Can you work these out from the model? Positions are in its coordinate system, mm. Give positions to 0.01 mm unless a question says otherwise; leave off trailing zeros. Order: outer loops, then holes, each group sorted by start corner. A loop starts at its lowest first (then second) coordinate and runs counter-clockwise, first axis right, second up. Notation, with made-up numbers: (44, 54) -> (70, 54) arc R36 cw to (70, 91) -> close; hole circle Ø3 at (61.25, 31.5). An arc over 180 degrees is marked (long way). Answer as a JSON object with one key per item and string values.
```python
from build123d import *

# Parameters (mm, degrees)
F0_W     = 25.4
F0_H     = 45.72
F0_W_2   = 6.35
F0_H_2   = 10.0076
F1_DEPTH = 3.175


with BuildPart() as f1:
    # F0 (on Top) → F1 (new body)
    with BuildSketch(Plane.XY):
        Polygon((-45.72, 76.2), (-76.2, 76.2), (-76.2, 45.72), (-73.025, 45.72), (-73.025, 15.24), (-76.2, 15.24), (-76.2, -15.24), (-73.025, -15.24), (-73.025, -45.72), (-76.2, -45.72), (-76.2, -76.2), (-45.72, -76.2), (-45.72, -73.025), (-15.24, -73.025), (-15.24, -76.2), (15.24, -76.2), (15.24, -73.025), (45.72, -73.025), (45.72, -76.2), (76.2, -76.2), (76.2, -45.72), (73.025, -45.72), (73.025, -15.24), (76.2, -15.24), (76.2, 15.24), (73.025, 15.24), (73.025, 45.72), (76.2, 45.72), (76.2, 76.2), (45.72, 76.2), (45.72, 73.025), (15.24, 73.025), (15.24, 76.2), (-15.24, 76.2), (-15.24, 73.025), (-45.72, 73.025), align=None)
        with Locations((-38.1, -38.1)):
            Rectangle(F0_W, F0_H, mode=Mode.SUBTRACT)
        with Locations((0, -38.1)):
            Rectangle(F0_W_2, F0_H_2, mode=Mode.SUBTRACT)
        with Locations((38.1, -38.1)):
            Rectangle(F0_W, F0_H, mode=Mode.SUBTRACT)
        with Locations((-38.1, 38.1)):
            Rectangle(F0_W, F0_H, mode=Mode.SUBTRACT)
        with Locations((0, 38.1)):
            Rectangle(F0_W_2, F0_H_2, mode=Mode.SUBTRACT)
        with Locations((38.1, 38.1)):
            Rectangle(F0_W, F0_H, mode=Mode.SUBTRACT)
    extrude(amount=F1_DEPTH)


solid = f1.part
```
1. If we section it at C-C on x = 42.5: Please give me the cut outline in (y, z) (3 decimals).
Worked answers:
{"outline": "(-73.025, 0) -> (-60.96, 0) -> (-60.96, 3.175) -> (-73.025, 3.175) -> close; (-15.24, 0) -> (15.24, 0) -> (15.24, 3.175) -> (-15.24, 3.175) -> close; (60.96, 0) -> (73.025, 0) -> (73.025, 3.175) -> (60.96, 3.175) -> close"}
2. If we section it at D-D on z = 1.6: Count the separate pieces of the cut face and the enclosed holes in it, then the cut area to 3 significant figures.
Worked answers:
{"separate pieces": "1", "enclosed holes": "6", "area": "17,700 mm²"}
3. Please list where these lines run through material, in increasing order: L1, parallel to X at y = 15.5, z = 2.6 (3 decimals); L2, parallel to X at y = -60, z = 0.9; L3, parallel to Y at x = 33, z = 2.8 (3 decimals).
Worked answers:
{"L1": "-73.025 to -50.8, -25.4 to 25.4, 50.8 to 73.025", "L2": "-76.2 to -50.8, -25.4 to 25.4, 50.8 to 76.2", "L3": "-73.025 to -60.96, -15.24 to 15.24, 60.96 to 73.025"}
4. If we section it at A-A on y = 41: Please give me the cut outline in (x, z) (3 decimals).
Worked answers:
{"outline": "(-73.025, 0) -> (-50.8, 0) -> (-50.8, 3.175) -> (-73.025, 3.175) -> close; (-25.4, 0) -> (-3.175, 0) -> (-3.175, 3.175) -> (-25.4, 3.175) -> close; (3.175, 0) -> (25.4, 0) -> (25.4, 3.175) -> (3.175, 3.175) -> close; (50.8, 0) -> (73.025, 0) -> (73.025, 3.175) -> (50.8, 3.175) -> close"}
5. Will these pins go through, and if not, where does the flat tip stop? pin 1 Ø1 at (y, z) = (-41, 2) entering from +X (3 decimals); pin 2 Ø1 at (x, z) = (-38, 1) entering from +Y (3 decimals); pin 3 Ø1 at (x, z) = (-33, 1) entering from -Y (3 decimals).
Worked answers:
{"pin 1": "x = 73.025", "pin 2": "y = 73.025", "pin 3": "y = -73.025"}
6. If we section it at B-B on y = 57: Please give me the cut outline in (x, z) (3 decimals), then the cut area to 3 significant figures.
Worked answers:
{"outline": "(-76.2, 0) -> (-50.8, 0) -> (-50.8, 3.175) -> (-76.2, 3.175) -> close; (-25.4, 0) -> (25.4, 0) -> (25.4, 3.175) -> (-25.4, 3.175) -> close; (50.8, 0) -> (76.2, 0) -> (76.2, 3.175) -> (50.8, 3.175) -> close", "area": "323 mm²"}
